Work out the finished part from the listing and answer in its coordinate system (mm). Face numbers are marked on the shaded views. A direction names the side the tool comes from. Give positions to 0.01 mm unless a question says otherwise; leave off trailing zeros. Loops run counter-clockwise (first coordinate to the right, second up) from the corner with the lowest first, then second, coordinate; pieces in that order, holes last. Notation, with made-up numbers: (65, 41) - (102, 41) arc R12 ccw to (102, 57) - close; hole circle Ø9 at (76, -11.5). An arc over 180 degrees is marked (long way). One line per item, written item: value.
from build123d import *

# Parameters (mm, degrees)
F1_W      = 5
F1_H      = 7.2
F1_H_2    = 6
F1_H_3    = 4
F1_W_2    = 23.3
F3_DEPTH  = 8.5
F0_W      = 23.3
F0_H      = 4
F4_DEPTH  = 23.2
F5_DEPTH  = 18.1
F6_START  = 4.3
F0_R      = 0.85
F6_DEPTH  = 20.7
F0_R_2    = 3.8
F7_DEPTH  = 5
F9_DEPTH  = 2.5
F10_DEPTH = 27.6


with BuildPart() as f3:
    # F1 (on Front) → F3 (new body, symmetric)
    with BuildSketch(Plane.XZ):
        with Locations((-14.15, 13.6)):
            Rectangle(F1_W, F1_H)
        with Locations((-14.15, 20.2)):
            Rectangle(F1_W, F1_H_2)
        with Locations((-14.15, 7)):
            Rectangle(F1_W, F1_H_2)
        with Locations((-14.15, 2)):
            Rectangle(F1_W, F1_H_3)
        with Locations((0, 2)):
            Rectangle(F1_W_2, F1_H_3)
        with Locations((14.15, 2)):
            Rectangle(F1_W, F1_H_3)
        with Locations((14.15, 7)):
            Rectangle(F1_W, F1_H_2)
        with Locations((14.15, 13.6)):
            Rectangle(F1_W, F1_H)
        with Locations((14.15, 20.2)):
            Rectangle(F1_W, F1_H_2)
    extrude(amount=F3_DEPTH, both=True)

    # F0 (on Top) → F4 (join)
    with BuildSketch(Plane.XY):
        with Locations((0, 6.5)):
            Rectangle(F0_W, F0_H)
    extrude(amount=F4_DEPTH)

    # F2 (on Right) → F5 (cut, symmetric)
    with BuildSketch(Plane.YZ):
        with BuildLine():
            Line((-8.5, 17.2), (-8.5, 10))
            Line((-8.5, 10), (3.5396314061, 10))
            ThreePointArc((3.5396314061, 10), (2.8089650426, 10.8020152096), (1.9224991399, 11.4275389379))
            Line((1.9224991399, 11.4275389379), (-5.9224991399, 15.7724610621))
            ThreePointArc((-5.9224991399, 15.7724610621), (-6.8089650426, 16.3979847904), (-7.5396314061, 17.2))
            Line((-7.5396314061, 17.2), (-8.5, 17.2))
        make_face()
        with BuildLine():
            Line((-8.5, 20.1464178425), (-8.5, 17.2))
            Line((-8.5, 17.2), (-7.5396314061, 17.2))
            ThreePointArc((-7.5396314061, 17.2), (-8.2538488107, 18.5969271247), (-8.5, 20.1464178425))
        make_face()
        with BuildLine():
            Line((-8.5, 10), (-8.5, 4))
            Line((-8.5, 4), (4.5, 4))
            Line((4.5, 4), (4.5, 7.0535821575))
            ThreePointArc((4.5, 7.0535821575), (4.2538488107, 8.6030728753), (3.5396314061, 10))
            Line((3.5396314061, 10), (-8.5, 10))
        make_face()
    extrude(amount=F5_DEPTH, both=True, mode=Mode.SUBTRACT)

    # F0 (on Top) → F6 (cut)
    with BuildSketch(Plane.XY.offset(F6_START)):
        with Locations((14.15, -2)):
            Circle(F0_R)
        with Locations((-14.15, -2)):
            Circle(F0_R)
    extrude(amount=F6_DEPTH, mode=Mode.SUBTRACT)

    # F0 (on Top) → F7 (join)
    with BuildSketch(Plane.XY):
        with Locations((-5.75, -2.2)):
            Circle(F0_R_2)
    extrude(amount=-F7_DEPTH)

    # F8 (on face) → F9 (join)
    with BuildSketch(Plane(origin=(0, 8.5, 0), x_dir=(-1, 0, 0), z_dir=(0, 1, 0))):
        with BuildLine():
            ThreePointArc((-7.95, 20.3), (-14.1018289963, 17.7518289963), (-16.65, 11.6))
            ThreePointArc((-16.65, 11.6), (-14.1018289963, 5.4481710037), (-7.95, 2.9))
            ThreePointArc((-7.95, 2.9), (-3.2863104735, 4.2556143892), (-0.075992126, 7.9))
            Line((-0.075992126, 7.9), (-7.95, 7.9))
            ThreePointArc((-7.95, 7.9), (-11.65, 11.6), (-7.95, 15.3))
            Line((-7.95, 15.3), (-0.075992126, 15.3))
            ThreePointArc((-0.075992126, 15.3), (-3.2863104735, 18.9443856108), (-7.95, 20.3))
        make_face()
        with BuildLine():
            Line((-7.95, 2.9), (16.65, 2.9))
            Line((16.65, 2.9), (16.65, 20.3))
            Line((16.65, 20.3), (-7.95, 20.3))
            ThreePointArc((-7.95, 20.3), (-3.2863104735, 18.9443856108), (-0.075992126, 15.3))
            Line((-0.075992126, 15.3), (8.35, 15.3))
            Line((8.35, 15.3), (8.35, 7.9))
            Line((8.35, 7.9), (-0.075992126, 7.9))
            ThreePointArc((-0.075992126, 7.9), (-3.2863104735, 4.2556143892), (-7.95, 2.9))
        make_face()
    extrude(amount=F9_DEPTH)

    # F8 (on face) → F10 (cut)
    with BuildSketch(Plane(origin=(0, 8.5, 0), x_dir=(-1, 0, 0), z_dir=(0, 1, 0))):
        with BuildLine():
            ThreePointArc((-5.85, 11.6), (-6.4650757595, 13.0849242405), (-7.95, 13.7))
            Line((-7.95, 13.7), (-7.95, 9.5))
            ThreePointArc((-7.95, 9.5), (-6.4650757595, 10.1150757595), (-5.85, 11.6))
        make_face()
        with BuildLine():
            Line((-7.95, 9.5), (-7.95, 13.7))
            ThreePointArc((-7.95, 13.7), (-10.05, 11.6), (-7.95, 9.5))
        make_face()
    extrude(amount=-F10_DEPTH, mode=Mode.SUBTRACT)


solid = f3.part
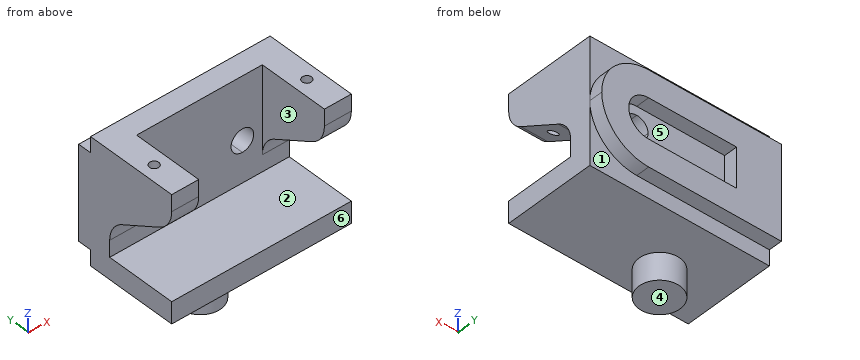
1. Flat-ended cylindrical pins translate along their axes: pin 1 Ø1.4 at (x, y) = (14.15, -2) entering from -Z; pin 2 Ø3 at (x, z) = (1, 15.5) entering from -Y; pin 3 Ø2 at (x, y) = (-8, 10.5) entering from +Z. Find the tip coordinate at first contact, or state that the pin passes through.
Output:
pin 1: stops at z = 0
pin 2: stops at y = 4.5
pin 3: stops at z = 20.3
2. Section B-B (x = -5.75) is taken. Write down the section's boundary in (y, z).
Output:
outline: (-8.5, 0) - (-6, 0) - (-6, -5) - (1.6, -5) - (1.6, 0) - (8.5, 0) - (8.5, 2.9) - (11, 2.9) - (11, 7.9) - (8.5, 7.9) - (8.5, 15.3) - (11, 15.3) - (11, 20.3) - (8.5, 20.3) - (8.5, 23.2) - (4.5, 23.2) - (4.5, 4) - (-8.5, 4) - close
3. The mould has two halves that part along Z. Classify the marked faces 4, 5 and 6: released by +Z, released by -Z, zero draft, split by the parting line, or undercut.
Output:
face 4: released by -Z
face 5: undercut
face 6: zero draft
4. Find the intervals of material crossed by line 1 along X through (y, z) = (-2, 15.75); line 2 along Z through (x, y) = (-7, 10.25); line 3 along X through (y, z) = (1.25, 17), in increasing order.
Output:
line 1: x = -16.65 to -15, -13.3 to -11.65, 11.65 to 13.3, 15 to 16.65
line 2: z = 2.9 to 7.9, 15.3 to 20.3
line 3: x = -16.65 to -11.65, 11.65 to 16.65
5. Section A-A (y = 9.5) is taken. Write down the section's boundary in (x, z), and give its area (3 significant figures).
Output:
outline: (-16.65, 2.9) - (7.95, 2.9) arc R8.7 ccw to (7.95, 20.3) - (-16.65, 20.3) - close; hole (-8.35, 7.9) - (7.95, 7.9) arc R3.7 ccw to (7.95, 15.3) - (-8.35, 15.3) - close
area: 405 mm²
6. Section D-D (x = -14.15) is taken. Write down the section's boundary in (y, z), and give its area (3 significant figures).
Output:
outline: (-8.5, 0) - (8.5, 0) - (8.5, 2.9) - (11, 2.9) - (11, 20.3) - (8.5, 20.3) - (8.5, 23.2) - (-1.15, 23.2) - (-1.15, 13.13) - (1.92, 11.43) arc R5 cw to (4.5, 7.05) - (4.5, 4) - (-8.5, 4) - close; (-8.5, 20.15) arc R5 ccw to (-5.92, 15.77) - (-2.85, 14.07) - (-2.85, 23.2) - (-8.5, 23.2) - close
area: 297 mm²
7. Section C-C (y = -4.5) is taken. Write down the section's boundary in (x, z), and give its area (3 significant figures).
Output:
outline: (-16.65, 0) - (-8.77, 0) - (-8.77, -5) - (-2.73, -5) - (-2.73, 0) - (16.65, 0) - (16.65, 4) - (-16.65, 4) - close; (-16.65, 14.98) - (-11.65, 14.98) - (-11.65, 23.2) - (-16.65, 23.2) - close; (11.65, 14.98) - (16.65, 14.98) - (16.65, 23.2) - (11.65, 23.2) - close
area: 246 mm²
8. For the marked faces 1, 2 and 3, determine the directions among +Z, -Z, +X, -X, +Y, -Y from which every point of the face is accessible in a straight line to the end or side of a thin tool.
Output:
face 1: -Z, +X, +Y
face 2: +X, -X, -Y
face 3: +Z, -Y
